For this review, use the dimensioned drawing (mm, ordinates from the lowest corner) and the shaded views. Coordinates: 2 decimals unless noted, no trailing zeros. Loops run counter-clockwise (first coordinate to the right, second up) from the corner with the lowest first, then second, coordinate; pieces in that order, holes last. Notation, with made-up numbers: M 76,28.5 L 125,28.5 A30 ccw 125,50.5 Z; hole C 16,-39 d6. An arc over 180 degrees is marked long. One line per item, written item: value.
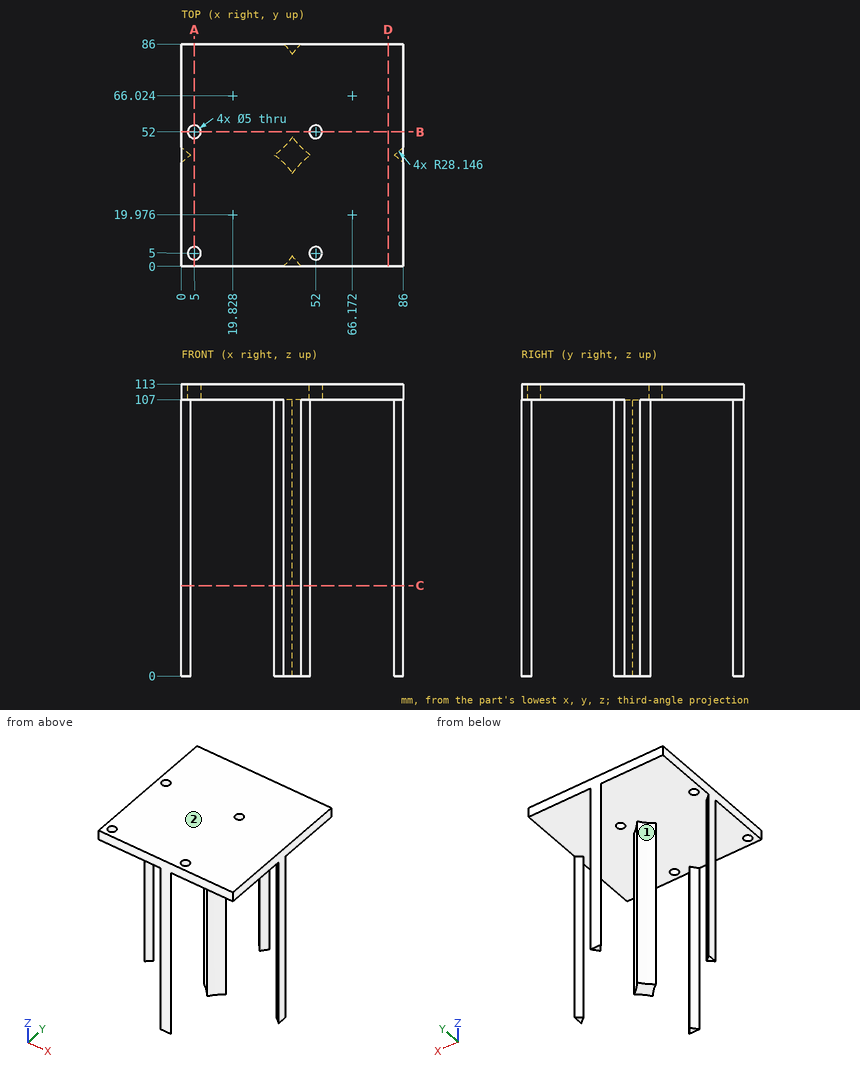
(1) Insertion check: pin 1 (4 mm diameter, centred on x = 50.5, y = 17, fed in from -Z); pin 2 (4.5 mm diameter, centred on x = 5, y = 5, fed in from +Z); pin 3 (6 mm diameter, centred on x = 50.5, z = 43.5, fed in from +Y). Each pin has a flat end and moves straight along its axis. Give the tip position at first contact, or say it passes through.
Reply:
pin 1: stops at z = 107
pin 2: passes through
pin 3: stops at y = 44.96
(2) We need section A-A on x = 5. State the section outline as (y, z) points, then the cut area to 3 significant figures.
Reply:
outline: M 0,107 L 2.5,107 L 2.5,113 L 0,113 Z; M 7.5,107 L 49.5,107 L 49.5,113 L 7.5,113 Z; M 54.5,107 L 86,107 L 86,113 L 54.5,113 Z
area: 456 mm2
(3) To check wall thickness, follow line 1 along Y through (x, z) = (52, 109); line 2 along Y through (x, z) = (42, 105.5) (1 decimal); line 3 along Z through (x, y) = (17, 59). State the ranges of each line that lie inside material, in increasing order. Write a range as [from, to].
Reply:
line 1: y = [0, 2.5], [7.5, 49.5], [54.5, 86]
line 2: y = [0, 2.6], [37.3, 48.7], [83.4, 86]
line 3: z = [107, 113]
(4) Mouldability with a two-part tool opening along X and no side actions: class the marked faces 1 and 2 as released by +X, released by -X, zero draft, split by the parting line, or undercut.
Reply:
face 1: undercut
face 2: zero draft
(5) We need section D-D on x = 80. State the section outline as (y, z) points, then the cut area to 3 significant figures.
Reply:
outline: M 0,107 L 86,107 L 86,113 L 0,113 Z
area: 516 mm2
(6) We need section C-C on z = 35. State the section outline as (x, y) points.
Reply:
outline: M 0,39.95 A28.15 cw 3.64,43 A28.15 cw 0,46.05 Z; M 36.02,43 A28.15 cw 43,35.95 A28.15 cw 49.98,43 A28.15 cw 43,50.05 A28.15 cw Z; M 39.66,0 L 46.34,0 A28.15 cw 43,4 A28.15 cw Z; M 39.66,86 A28.15 cw 43,82 A28.15 cw 46.34,86 Z; M 82.36,43 A28.15 cw 86,39.95 L 86,46.05 A28.15 cw Z
